Part model, mm, in its own coordinate system. A direction names the side the tool comes from. Round coordinates to 2 decimals unless told otherwise and drop trailing zeros. Loops run counter-clockwise (first coordinate to the right, second up) from the corner with the lowest first, then second, coordinate; pieces in that order, holes last.
from build123d import *

# Parameters (mm, degrees)
SKETCH1_W              = 202
SKETCH1_H              = 74
BOSS_EXTRUDE1_DEPTH    = 1.6002
M3_CLEARANCE_HOLE1_D   = 3.4
SKETCH3_W              = 202
SKETCH3_H              = 2.5875
BOSS_EXTRUDE2_DEPTH    = 38
SKETCH6_W              = 35
SKETCH6_H              = 2.5875
SKETCH6_W_2            = 26
BOSS_EXTRUDE3_DEPTH    = 38
SKETCH7_W              = 2.5875
SKETCH7_H              = 72
BOSS_EXTRUDE4_DEPTH    = 38
SKETCH8_W              = 65
SKETCH8_H              = 45
BOSS_EXTRUDE5_DEPTH    = 1.6002
SKETCH9_W              = 65
SKETCH9_H              = 38
BOSS_EXTRUDE6_DEPTH    = 2.5875
SKETCH10_W             = 2.5875
SKETCH10_H             = 43
SKETCH10_W_2           = 64
SKETCH10_H_2           = 2.5875
BOSS_EXTRUDE7_DEPTH    = 38
CUT_EXTRUDE1_DEPTH     = 36.3998
CONVERT_SOLID1_START   = -101
CONVERT_SOLID1_DEPTH   = 202
CONVERT_SOLID1_START_2 = -166
CONVERT_SOLID1_2_DEPTH = 64
CONVERT_SOLID1_START_3 = -102
CONVERT_SOLID1_3_DEPTH = 36
CONVERT_SOLID1_START_4 = 75
CONVERT_SOLID1_4_DEPTH = 26
CONVERT_SOLID1_START_5 = -7
CONVERT_SOLID1_5_DEPTH = 43
CONVERT_SOLID1_START_6 = -36
CONVERT_SOLID1_6_DEPTH = 29
CONVERT_SOLID1_7_DEPTH = 267
CONVERT_SOLID1_8_DEPTH = 64
CONVERT_SOLID1_9_DEPTH = 72
FILLET1_R              = 4


# Read off the part's stored shape, not the designer's step: Convert-Solid1
with BuildPart() as part:
    # Sketch1 → Boss-Extrude1 (new body)
    with BuildSketch(Plane.XY):
        Rectangle(SKETCH1_W, SKETCH1_H)
    extrude(amount=BOSS_EXTRUDE1_DEPTH)

    # M3 Clearance Hole1 (through all)
    with Locations(Plane.XY.offset(1.6002)):
        with Locations((-96.5, 17.5), (95.5, -17.5), (-96.5, -17.5), (95.5, 17.5)):
            Hole(M3_CLEARANCE_HOLE1_D / 2)

    # Sketch3 → Boss-Extrude2 (add)
    with BuildSketch(Plane.XY):
        with Locations((0, -38.29375)):
            Rectangle(SKETCH3_W, SKETCH3_H)
    extrude(amount=BOSS_EXTRUDE2_DEPTH)

    # Sketch6 → Boss-Extrude3 (add)
    with BuildSketch(Plane.XY):
        with Locations((-83.5, 38.29375)):
            Rectangle(SKETCH6_W, SKETCH6_H)
        with Locations((88, 38.29375)):
            Rectangle(SKETCH6_W_2, SKETCH6_H)
    extrude(amount=BOSS_EXTRUDE3_DEPTH)

    # Sketch7 → Boss-Extrude4 (add)
    with BuildSketch(Plane.XY):
        with Locations((102.29375, 0)):
            Rectangle(SKETCH7_W, SKETCH7_H)
    extrude(amount=BOSS_EXTRUDE4_DEPTH)

    # Sketch8 → Boss-Extrude5 (add)
    with BuildSketch(Plane.XY):
        with Locations((-133.5, 14.5)):
            Rectangle(SKETCH8_W, SKETCH8_H)
    extrude(amount=BOSS_EXTRUDE5_DEPTH)

    # Sketch9 → Boss-Extrude6 (add)
    with BuildSketch(Plane(origin=(0, 37, 0), x_dir=(1, 0, 0), z_dir=(0, 1, 0))):
        with Locations((-133.5, -19)):
            Rectangle(SKETCH9_W, SKETCH9_H)
    extrude(amount=BOSS_EXTRUDE6_DEPTH)

    # Sketch10 → Boss-Extrude7 (add)
    with BuildSketch(Plane.XY):
        with Locations((-167.29375, 14.5)):
            Rectangle(SKETCH10_W, SKETCH10_H)
        with Locations((-134, -9.29375)):
            Rectangle(SKETCH10_W_2, SKETCH10_H_2)
    extrude(amount=BOSS_EXTRUDE7_DEPTH)

    # Sketch15 → Cut-Extrude1 (cut)
    with BuildSketch(Plane.XY.offset(38)):
        Polygon((102, 38), (-167, 38), (-167, -9), (-102, -9), (-102, -38), (102, -38), align=None)
    extrude(amount=-CUT_EXTRUDE1_DEPTH, mode=Mode.SUBTRACT)

    # Convert-Solid1 outline → Convert-Solid1 (add)
    with BuildSketch(Plane.YZ.offset(CONVERT_SOLID1_START)):
        with BuildLine():
            Line((-38, 1.6002), (-37.238, 1.6002))
            ThreePointArc((-37.238, 1.6002), (-37.776815367, 1.823384633), (-38, 2.3622))
            Line((-38, 2.3622), (-38, 1.6002))
        make_face()
        with BuildLine():
            Line((-39.5875, 2.117580723), (-39.5875, 38))
            Line((-39.5875, 38), (-39.6002, 38))
            Line((-39.6002, 38), (-39.6002, 2.3622))
            ThreePointArc((-39.6002, 2.3622), (-39.597022863, 2.239725635), (-39.5875, 2.117580723))
        make_face()
    extrude(amount=CONVERT_SOLID1_DEPTH)

    # Convert-Solid1 2 outline → Convert-Solid1 2 (add)
    with BuildSketch(Plane.YZ.offset(CONVERT_SOLID1_START_2)):
        with BuildLine():
            ThreePointArc((-10.6002, 2.3622), (-10.597022863, 2.239725635), (-10.5875, 2.117580723))
            Line((-10.5875, 2.117580723), (-10.5875, 38))
            Line((-10.5875, 38), (-10.6002, 38))
            Line((-10.6002, 38), (-10.6002, 2.3622))
        make_face()
        with BuildLine():
            Line((-9, 2.3622), (-9, 1.6002))
            Line((-9, 1.6002), (-8.238, 1.6002))
            ThreePointArc((-8.238, 1.6002), (-8.776815367, 1.823384633), (-9, 2.3622))
        make_face()
        with BuildLine():
            ThreePointArc((38, 2.3622), (37.776815367, 1.823384633), (37.238, 1.6002))
            Line((37.238, 1.6002), (38, 1.6002))
            Line((38, 1.6002), (38, 2.3622))
        make_face()
        with BuildLine():
            Line((39.5875, 38), (39.5875, 2.117580723))
            ThreePointArc((39.5875, 2.117580723), (39.597022863, 2.239725635), (39.6002, 2.3622))
            Line((39.6002, 2.3622), (39.6002, 38))
            Line((39.6002, 38), (39.5875, 38))
        make_face()
    extrude(amount=CONVERT_SOLID1_2_DEPTH)

    # Convert-Solid1 3 outline → Convert-Solid1 3 (add)
    with BuildSketch(Plane.YZ.offset(CONVERT_SOLID1_START_3)):
        with BuildLine():
            ThreePointArc((38, 2.3622), (37.776815367, 1.823384633), (37.238, 1.6002))
            Line((37.238, 1.6002), (38, 1.6002))
            Line((38, 1.6002), (38, 2.3622))
        make_face()
        with BuildLine():
            Line((39.5875, 38), (39.5875, 2.117580723))
            ThreePointArc((39.5875, 2.117580723), (39.597022863, 2.239725635), (39.6002, 2.3622))
            Line((39.6002, 2.3622), (39.6002, 38))
            Line((39.6002, 38), (39.5875, 38))
        make_face()
    extrude(amount=CONVERT_SOLID1_3_DEPTH)

    # Convert-Solid1 4 outline → Convert-Solid1 4 (add)
    with BuildSketch(Plane.YZ.offset(CONVERT_SOLID1_START_4)):
        with BuildLine():
            ThreePointArc((38, 2.3622), (37.776815367, 1.823384633), (37.238, 1.6002))
            Line((37.238, 1.6002), (38, 1.6002))
            Line((38, 1.6002), (38, 2.3622))
        make_face()
        with BuildLine():
            Line((39.5875, 38), (39.5875, 2.117580723))
            ThreePointArc((39.5875, 2.117580723), (39.597022863, 2.239725635), (39.6002, 2.3622))
            Line((39.6002, 2.3622), (39.6002, 38))
            Line((39.6002, 38), (39.5875, 38))
        make_face()
    extrude(amount=CONVERT_SOLID1_4_DEPTH)

    # Convert-Solid1 5 outline → Convert-Solid1 5 (add)
    with BuildSketch(Plane(origin=(0, 0, 0), x_dir=(1, 0, 0), z_dir=(0, 1, 0)).offset(CONVERT_SOLID1_START_5)):
        with BuildLine():
            ThreePointArc((-167, -2.3622), (-166.776815367, -1.823384633), (-166.238, -1.6002))
            Line((-166.238, -1.6002), (-167, -1.6002))
            Line((-167, -1.6002), (-167, -2.3622))
        make_face()
        with BuildLine():
            Line((102, -1.6002), (101.238, -1.6002))
            ThreePointArc((101.238, -1.6002), (101.776815367, -1.823384633), (102, -2.3622))
            Line((102, -2.3622), (102, -1.6002))
        make_face()
        with BuildLine():
            Line((-168.6002, -38), (-168.5875, -38))
            Line((-168.5875, -38), (-168.5875, -2.117580723))
            ThreePointArc((-168.5875, -2.117580723), (-168.597022863, -2.239725635), (-168.6002, -2.3622))
            Line((-168.6002, -2.3622), (-168.6002, -38))
        make_face()
        with BuildLine():
            Line((103.5875, -2.117580723), (103.5875, -38))
            Line((103.5875, -38), (103.6002, -38))
            Line((103.6002, -38), (103.6002, -2.3622))
            ThreePointArc((103.6002, -2.3622), (103.597022863, -2.239725635), (103.5875, -2.117580723))
        make_face()
    extrude(amount=CONVERT_SOLID1_5_DEPTH)

    # Convert-Solid1 6 outline → Convert-Solid1 6 (add)
    with BuildSketch(Plane(origin=(0, 0, 0), x_dir=(1, 0, 0), z_dir=(0, 1, 0)).offset(CONVERT_SOLID1_START_6)):
        with BuildLine():
            Line((102, -1.6002), (101.238, -1.6002))
            ThreePointArc((101.238, -1.6002), (101.776815367, -1.823384633), (102, -2.3622))
            Line((102, -2.3622), (102, -1.6002))
        make_face()
        with BuildLine():
            Line((103.5875, -2.117580723), (103.5875, -38))
            Line((103.5875, -38), (103.6002, -38))
            Line((103.6002, -38), (103.6002, -2.3622))
            ThreePointArc((103.6002, -2.3622), (103.597022863, -2.239725635), (103.5875, -2.117580723))
        make_face()
    extrude(amount=CONVERT_SOLID1_6_DEPTH)

    # Convert-Solid1 7 outline → Convert-Solid1 7 (cut)
    with BuildSketch(Plane.YZ.offset(CONVERT_SOLID1_START_2)):
        with BuildLine():
            Line((-10.5875, 2.117580723), (-10.5875, 1.6002))
            Line((-10.5875, 1.6002), (-10.473921475, 1.6002))
            ThreePointArc((-10.473921475, 1.6002), (-10.545258813, 1.855696681), (-10.5875, 2.117580723))
        make_face()
        with BuildLine():
            Line((-39.5875, 0), (-37.238, 0))
            ThreePointArc((-37.238, 0), (-38.81947861, 0.607516482), (-39.5875, 2.117580723))
            Line((-39.5875, 2.117580723), (-39.5875, 0))
        make_face()
        with BuildLine():
            ThreePointArc((39.5875, 2.117580723), (38.81947861, 0.607516482), (37.238, 0))
            Line((37.238, 0), (39.5875, 0))
            Line((39.5875, 0), (39.5875, 2.117580723))
        make_face()
    extrude(amount=CONVERT_SOLID1_7_DEPTH, mode=Mode.SUBTRACT)

    # Convert-Solid1 8 outline → Convert-Solid1 8 (cut)
    with BuildSketch(Plane.YZ.offset(CONVERT_SOLID1_START_2)):
        with BuildLine():
            Line((-10.473921475, 1.6002), (-10.5875, 1.6002))
            Line((-10.5875, 1.6002), (-10.5875, 0))
            Line((-10.5875, 0), (-8.238, 0))
            ThreePointArc((-8.238, 0), (-9.612771334, 0.441264649), (-10.473921475, 1.6002))
        make_face()
    extrude(amount=CONVERT_SOLID1_8_DEPTH, mode=Mode.SUBTRACT)

    # Convert-Solid1 9 outline → Convert-Solid1 9 (cut)
    with BuildSketch(Plane(origin=(0, 0, 0), x_dir=(1, 0, 0), z_dir=(0, 1, 0)).offset(CONVERT_SOLID1_START_6)):
        with BuildLine():
            Line((-168.5875, 0), (-168.5875, -2.117580723))
            ThreePointArc((-168.5875, -2.117580723), (-167.81947861, -0.607516482), (-166.238, 0))
            Line((-166.238, 0), (-168.5875, 0))
        make_face()
        with BuildLine():
            ThreePointArc((101.238, 0), (102.81947861, -0.607516482), (103.5875, -2.117580723))
            Line((103.5875, -2.117580723), (103.5875, 0))
            Line((103.5875, 0), (101.238, 0))
        make_face()
    extrude(amount=CONVERT_SOLID1_9_DEPTH, mode=Mode.SUBTRACT)

    # Fillet1
    fillet1_edges = [part.edges().sort_by_distance(p)[0] for p in [
        (75, 38.8001, 38),
        (101, 38.8001, 38),
        (102.8001, 36, 38),
        (102.8001, -36, 38),
        (101, -38.8001, 38),
        (-101, -38.8001, 38),
        (-102, -9.8001, 38),
        (-166, -9.8001, 38),
        (-167.8001, -7, 38),
        (-167.8001, 36, 38),
        (-166, 38.8001, 38),
        (-66, 38.8001, 38),
    ]]
    fillet(fillet1_edges, radius=FILLET1_R)


solid = part.part
1) Tool access for faces 1 (the face through (-134, -10.6, 20)), 2 (the face through (-134, -9, 20)), 3 (the face through (-34, 1, 0)), 4 (the face through (-167, 15, 20)), 5 (the face through (-115, 38, 20)): list every direction of +Z, -Z, +X, -X, +Y, -Y with a clear straight run to the whole face (end or side of a thin tool).
Values:
face 1: +Z, -Z, -X, -Y
face 2: +Z, -X
face 3: -Z, +X, -X, +Y, -Y
face 4: +Z, +Y, -Y
face 5: +Z, +X, -X
2) Slice it at A-A, the plane z = 23. Give the cut face in (x, y), then the cut area to 3 significant figures.
Values:
outline: (-168.6, -7) - (-167, -7) - (-167, 36) - (-168.6, 36) - close; (-166, -10.6) - (-102, -10.6) - (-102, -9) - (-166, -9) - close; (-166, 38) - (-66, 38) - (-66, 39.6) - (-166, 39.6) - close; (-101, -39.6) - (101, -39.6) - (101, -38) - (-101, -38) - close; (75, 38) - (101, 38) - (101, 39.6) - (75, 39.6) - close; (102, -36) - (103.6, -36) - (103.6, 36) - (102, 36) - close
area: 811 mm2
3) Mould opens along X. For faces 6 (the face through (102, -1, 20)), 7 (the face through (-117, 39.6, 20)), 8 (the face through (-168.6, 14, 20)), 9 (the face through (-34, 1, 1.6)) say: released by +X, released by -X, zero draft, split by the parting line, or undercut.
Values:
face 6: undercut
face 7: zero draft
face 8: released by -X
face 9: undercut
4) Drop flat-ended pins along their axis: pin 1 Ø4.5 at (x, y) = (-96.5, 17.5) entering from +Z; pin 2 Ø5 at (x, z) = (-27.5, 27) entering from +Y; pin 3 Ø10 at (y, z) = (-19, 21.5) entering from -X; pin 4 Ø8 at (x, y) = (23, -15) entering from -Z. Give the stop position or say it passes through.
Values:
pin 1: stops at z = 1.6
pin 2: stops at y = -38
pin 3: stops at x = 102
pin 4: stops at z = 0
5) Slice it at B-B, the plane x = -132.5. Give the cut face in (y, z), then the cut area to 3 significant figures.
Values:
outline: (-10.6, 2.36) arc R2.36 ccw to (-8.24, 0) - (37.24, 0) arc R2.36 ccw to (39.6, 2.36) - (39.6, 38) - (38, 38) - (38, 2.36) arc R0.76 cw to (37.24, 1.6) - (-8.24, 1.6) arc R0.76 cw to (-9, 2.36) - (-9, 38) - (-10.6, 38) - close
area: 195 mm2
6) Slice it at C-C, the plane y = 21.5. Give the cut face in (x, z), then the cut area to 3 significant figures.
Values:
outline: (-168.6, 2.36) arc R2.36 ccw to (-166.24, 0) - (101.24, 0) arc R2.36 ccw to (103.6, 2.36) - (103.6, 38) - (102, 38) - (102, 2.36) arc R0.76 cw to (101.24, 1.6) - (-166.24, 1.6) arc R0.76 cw to (-167, 2.36) - (-167, 38) - (-168.6, 38) - close
area: 550 mm2
7) Wall check: line 1 along Y through (x, z) = (95, 1); line 2 along X through (y, z) = (29.5, 30); line 3 along Y through (x, z) = (-136.5, 26). Give the ranges that are in metal, low to high.
Values:
line 1: y = -39.17 to -19.12, -15.88 to 15.88, 19.12 to 39.17
line 2: x = -168.6 to -167, 102 to 103.6
line 3: y = -10.6 to -9, 38 to 39.6
8) Slice it at D-D, the plane x = -26.5. Give the cut face in (y, z).
Values:
outline: (-39.6, 2.36) arc R2.36 ccw to (-37.24, 0) - (37, 0) - (37, 1.6) - (-37.24, 1.6) arc R0.76 cw to (-38, 2.36) - (-38, 38) - (-39.6, 38) - close
